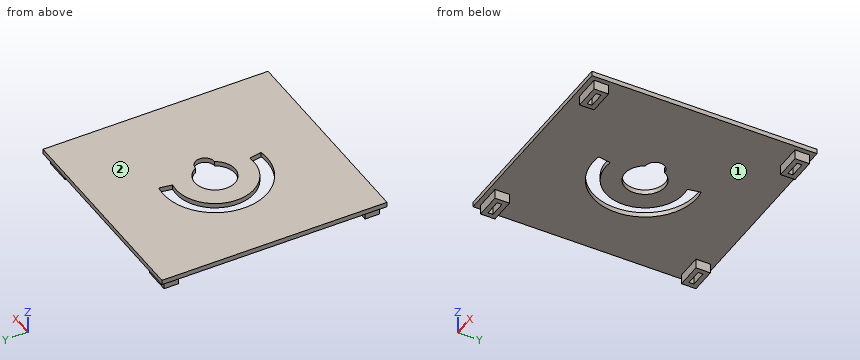
```python
from build123d import *

# Parameters (mm, degrees)
SKETCH1_W                 = 65.925
SKETCH1_H                 = 70
BOSS_EXTRUDE1_DEPTH       = 1.5
CUT_EXTRUDE1_REACH        = 137.268
SKETCH4_W                 = 8
SKETCH4_H                 = 4.5
SKETCH4_W_2               = 5
SKETCH4_H_2               = 1.5
BOSS_EXTRUDE2_DEPTH       = 3
MIRROR2_COPY_1_SKETCH_W   = 8
MIRROR2_COPY_1_SKETCH_H   = 4.5
MIRROR2_COPY_1_SKETCH_W_2 = 5
MIRROR2_COPY_1_SKETCH_H_2 = 1.5
MIRROR2_COPY_1_DEPTH      = 3
CUT_EXTRUDE2_DEPTH        = 136.334853235


with BuildPart() as part:
    # Sketch1 → Boss-Extrude1 (new body)
    with BuildSketch(Plane.XY):
        with Locations((88.1375, 25.25)):
            Rectangle(SKETCH1_W, SKETCH1_H)
    extrude(amount=BOSS_EXTRUDE1_DEPTH)

    # Sketch2 → Cut-Extrude1 (cut, up to next)
    with BuildSketch(Plane.XY.offset(1.5), mode=Mode.PRIVATE) as cut_extrude1_sk1:
        with BuildLine():
            Line((93.647490926, 22.3), (93.7375, 22.3))
            ThreePointArc((93.7375, 22.3), (96.6875, 25.25), (93.7375, 28.2))
            Line((93.7375, 28.2), (93.647490926, 28.2))
            ThreePointArc((93.647490926, 28.2), (81.8875, 25.25), (93.647490926, 22.3))
        make_face()
    cut_extrude1_tool1 = extrude(cut_extrude1_sk1.sketch, amount=-CUT_EXTRUDE1_REACH, mode=Mode.PRIVATE) & part.part
    add(cut_extrude1_tool1.solids().sort_by_distance((88.730915, 25.25, 1.5))[0], mode=Mode.SUBTRACT)

    # Sketch4 → Boss-Extrude2 (add)
    with BuildSketch(Plane(origin=(0, 0, 0), x_dir=(-1, 0, 0), z_dir=(0, 0, -1))):
        with Locations((-115.6, 56.5)):
            Rectangle(SKETCH4_W, SKETCH4_H)
        with Locations((-115.6, 56.5)):
            Rectangle(SKETCH4_W_2, SKETCH4_H_2, mode=Mode.SUBTRACT)
    boss_extrude2 = extrude(amount=BOSS_EXTRUDE2_DEPTH)

    # Mirror1: Boss-Extrude2 across plane
    add(boss_extrude2.mirror(Plane(origin=(88.1375, 0, 0), x_dir=(0, 0, 1), z_dir=(1, 0, 0))))

    # Mirror2: Boss-Extrude2 across plane
    add(boss_extrude2.mirror(Plane.ZX.offset(25.25)))

    # Mirror2 copy 1 sketch → Mirror2 copy 1 (add)
    with BuildSketch(Plane(origin=(176.275, 50.5, 0), x_dir=(1, 0, 0), z_dir=(0, 0, -1))):
        with Locations((-115.6, 56.5)):
            Rectangle(MIRROR2_COPY_1_SKETCH_W, MIRROR2_COPY_1_SKETCH_H)
        with Locations((-115.6, 56.5)):
            Rectangle(MIRROR2_COPY_1_SKETCH_W_2, MIRROR2_COPY_1_SKETCH_H_2, mode=Mode.SUBTRACT)
    extrude(amount=MIRROR2_COPY_1_DEPTH)

    # Sketch5 → Cut-Extrude2 (cut, through all)
    with BuildSketch(Plane.XY.offset(1.5)):
        with BuildLine():
            Line((90.254036985, 37.253477721), (90.948629695, 41.192708733))
            ThreePointArc((90.948629695, 41.192708733), (71.948849287, 25.25), (90.948629695, 9.307291267))
            Line((90.948629695, 9.307291267), (90.254036985, 13.246522279))
            ThreePointArc((90.254036985, 13.246522279), (75.948849287, 25.25), (90.254036985, 37.253477721))
        make_face()
    extrude(amount=-CUT_EXTRUDE2_DEPTH, mode=Mode.SUBTRACT)


solid = part.part
```
Check sheet for the modelled part. Datum: model origin and axes. Units: mm. Face numbers are marked on the shaded views. Give positions to 0.01 mm unless a question says otherwise; leave off trailing zeros. Order: outer loops, then holes, each group sorted by start corner. A loop starts at its lowest first (then second) coordinate and runs counter-clockwise, first axis right, second up. Notation, with made-up numbers: M 38,-6 L 46,-6 A29 cw 46,15 Z; hole C 1.25,-7.5 d8. An arc over 180 degrees is marked long. Answer in a Markdown table with one row per item.
1) Cross-section at B-B, the plane y = 25.25. Enter the section's corners in (x, z) (1 decimal), plus the area to 3 significant figures.
Filled sheet:
| item | result |
|---|---|
| outline | M 55.2,0 L 71.9,0 L 71.9,1.5 L 55.2,1.5 Z; M 75.9,0 L 81.9,0 L 81.9,1.5 L 75.9,1.5 Z; M 96.7,0 L 121.1,0 L 121.1,1.5 L 96.7,1.5 Z |
| area | 70.7 mm2 |
2) Thickness scan on L1, parallel to X at y = 25.25, z = 0.9 (1 decimal); L2, parallel to Y at x = 118, z = -1.8; L3, parallel to Y at x = 64, z = -1.2. Record the ranges inside material, lowest first. Write a range as [from, to].
Filled sheet:
| item | result |
|---|---|
| L1 | x = [55.2, 71.9], [75.9, 81.9], [96.7, 121.1] |
| L2 | y = [-8.25, -6.75], [-5.25, -3.75], [54.25, 55.75], [57.25, 58.75] |
| L3 | y = [-8.25, -3.75], [54.25, 58.75] |
3) Cross-section at A-A, the plane z = -1.55. Count the separate pieces of the cut face and the enclosed holes in it, plus the area to 3 significant figures.
Filled sheet:
| item | result |
|---|---|
| separate pieces | 4 |
| enclosed holes | 4 |
| area | 114 mm2 |
4) Release check for a two-part mould opening along Y. For the marked faces 1 and 2 record: +Y half, -Y half, draft (parallel to the pull), parting line (faces both ways), or undercut.
Filled sheet:
| item | result |
|---|---|
| face 1 | undercut |
| face 2 | draft |
5) Cross-section at C-C, the plane x = 83. Enter the section's corners in (y, z), plus the area to 3 significant figures.
Filled sheet:
| item | result |
|---|---|
| outline | M -9.75,0 L 9.9,0 L 9.9,1.5 L -9.75,1.5 Z; M 14.2,0 L 21.69,0 L 21.69,1.5 L 14.2,1.5 Z; M 28.81,0 L 36.3,0 L 36.3,1.5 L 28.81,1.5 Z; M 40.6,0 L 60.25,0 L 60.25,1.5 L 40.6,1.5 Z |
| area | 81.4 mm2 |
6) Cross-section at D-D, the plane x = 114. Enter the section's corners in (y, z), plus the area to 3 significant figures.
Filled sheet:
| item | result |
|---|---|
| outline | M -9.75,0 L -8.25,0 L -8.25,-3 L -6.75,-3 L -6.75,0 L -5.25,0 L -5.25,-3 L -3.75,-3 L -3.75,0 L 54.25,0 L 54.25,-3 L 55.75,-3 L 55.75,0 L 57.25,0 L 57.25,-3 L 58.75,-3 L 58.75,0 L 60.25,0 L 60.25,1.5 L -9.75,1.5 Z |
| area | 123 mm2 |
7) Gauge pin test, flat ends, axial feed: P1, Ø0.9, axis at x = 60, z = -1, coming from the +Y side; P2, Ø1.2, axis at y = -6, z = -1, coming from the +X side; P3, Ø0.9, axis at y = -5.5, z = -1, coming from the -X side (3 decimals). Record the tip position at first contact, or that the pin passes through.
Filled sheet:
| item | result |
|---|---|
| P1 | stops at y = 58.75 |
| P2 | stops at x = 119.6 |
| P3 | stops at x = 56.675 |
